```python
from build123d import *

# Parameters (mm, degrees)
ESQUISSE1_W        = 150
ESQUISSE1_H        = 50
ESQUISSE1_R        = 1
BOSS_EXTRU_4_DEPTH = 10
BOSS_EXTRU_5_DEPTH = 10


with BuildPart() as part:
    # Esquisse1 → Boss.-Extru.4 (new body)
    with BuildSketch(Plane(origin=(0, 0, -20), x_dir=(-1, 0, 0), z_dir=(0, 0, -1))):
        with Locations((11.141434162, -115.464178298)):
            Rectangle(ESQUISSE1_W, ESQUISSE1_H)
        with Locations((-43.858565838, -128.464178298)):
            Circle(ESQUISSE1_R, mode=Mode.SUBTRACT)
        with Locations((-43.858565838, -115.464178298)):
            Circle(ESQUISSE1_R, mode=Mode.SUBTRACT)
        with Locations((-33.858565838, -100.464178298)):
            Circle(ESQUISSE1_R, mode=Mode.SUBTRACT)
        with Locations((-8.858565838, -100.464178298)):
            Circle(ESQUISSE1_R, mode=Mode.SUBTRACT)
        with Locations((1.141434162, -115.464178298)):
            Circle(ESQUISSE1_R, mode=Mode.SUBTRACT)
        with Locations((1.141434162, -128.464178298)):
            Circle(ESQUISSE1_R, mode=Mode.SUBTRACT)
        with Locations((46.141434162, -123.464178298)):
            Circle(ESQUISSE1_R, mode=Mode.SUBTRACT)
        with Locations((46.141434162, -110.464178298)):
            Circle(ESQUISSE1_R, mode=Mode.SUBTRACT)
        with Locations((61.141434162, -100.464178298)):
            Circle(ESQUISSE1_R, mode=Mode.SUBTRACT)
        with Locations((76.141434162, -110.464178298)):
            Circle(ESQUISSE1_R, mode=Mode.SUBTRACT)
        with Locations((76.141434162, -123.464178298)):
            Circle(ESQUISSE1_R, mode=Mode.SUBTRACT)
    extrude(amount=BOSS_EXTRU_4_DEPTH)

    # Esquisse3 → Boss.-Extru.5 (add)
    with BuildSketch(Plane.XY.offset(-20)):
        Polygon((-1.141434162, -100.464178298), (-1.141434162, -90.464178298), (-21.141434162, -90.464178298), (-21.141434162, -140.464178298), (-11.141434162, -140.464178298), (-11.141434162, -100.464178298), align=None)
        Polygon((63.858565838, -140.464178298), (63.858565838, -90.464178298), (43.858565838, -90.464178298), (43.858565838, -100.464178298), (53.858565838, -100.464178298), (53.858565838, -140.464178298), align=None)
    extrude(amount=BOSS_EXTRU_5_DEPTH)


solid = part.part
```
Design review of the part built by this model. Coordinates are the model's own, in mm. A direction names the side the tool comes from. Coordinates: 2 decimals unless noted, no trailing zeros. Write each loop counter-clockwise with the first axis right and the second up, starting at its lowest first coordinate (ties: lowest second). Pieces come first, ordered by that corner, then holes.
1) Add section D-D (y = -107.5). Write out the cut boundary in (x, z), plus the area to 3 significant figures.
2) To check wall thickness, follow L1, parallel to X at y = -137.5, z = -19; L2, parallel to X at y = -92.5, z = -19.5; L3, parallel to Y at x = 53, z = -19.25. State the ranges of each line that lie inside material, in increasing order.
3) Add section A-A (z = -16.25). Write out the cut boundary in (x, y), plus the area to 3 significant figures.
4) Add section C-C (x = -6). Write out the cut boundary in (y, z), plus the area to 3 significant figures.
5) Add section B-B (y = -95). Write out the cut boundary in (x, z), plus the area to 3 significant figures.
6) Insertion check: pin 1 (11 mm diameter, centred on x = -5, z = -17, fed in from -Y); pin 2 (3 mm diameter, centred on x = -46.14, y = -123.46, fed in from +Z); pin 3 (5 mm diameter, centred on y = -127.5, z = -17, fed in from -X). Each pin has a flat end and moves straight along its axis. Give the tip position at first contact, or say it passes through.
7) Mouldability with a two-part tool opening along X and no side actions: class faces 1 (the flat face through (-21.141, -115, -15)), 2 (the flat face through (-1.141, -96, -15)), 3 (the flat face through (43.859, -95, -15)), 4 (the flat face through (-14, -110, -10)) as +X half, -X half, draft (parallel to the pull), parting line (faces both ways), or undercut.
8) Machinability: for faces 5 (the flat face through (-10, -90.464, -22)), 6 (the flat face through (-11.141, -121, -15)), 7 (the flat face through (-53, -115, -20)), which of the approach directions +Z, -Z, +X, -X, +Y, -Y give a long, thin tool a straight path to every point of the face, cutting with its end or side? Answer none if there is none.
Check result:
1. outline: (-86.14, -30) - (63.86, -30) - (63.86, -10) - (53.86, -10) - (53.86, -20) - (-11.14, -20) - (-11.14, -10) - (-21.14, -10) - (-21.14, -20) - (-86.14, -20) - close
1. area: 1,700 mm2
2. L1: x = -21.14 to -11.14, 53.86 to 63.86
2. L2: x = -21.14 to -1.14, 43.86 to 63.86
2. L3: y = -100.46 to -90.46
3. outline: (-21.14, -140.46) - (-11.14, -140.46) - (-11.14, -100.46) - (-1.14, -100.46) - (-1.14, -90.46) - (-21.14, -90.46) - close; (43.86, -100.46) - (53.86, -100.46) - (53.86, -140.46) - (63.86, -140.46) - (63.86, -90.46) - (43.86, -90.46) - close
3. area: 1,200 mm2
4. outline: (-140.46, -30) - (-90.46, -30) - (-90.46, -10) - (-100.46, -10) - (-100.46, -20) - (-140.46, -20) - close
4. area: 600 mm2
5. outline: (-86.14, -30) - (63.86, -30) - (63.86, -10) - (43.86, -10) - (43.86, -20) - (-1.14, -20) - (-1.14, -10) - (-21.14, -10) - (-21.14, -20) - (-86.14, -20) - close
5. area: 1,900 mm2
6. pin 1: stops at y = -140.46
6. pin 2: stops at z = -20
6. pin 3: stops at x = -21.14
7. face 1: -X half
7. face 2: undercut
7. face 3: undercut
7. face 4: draft
8. face 5: +Z, -Z, +X, -X, +Y
8. face 6: +Z, -Y
8. face 7: +Z, -X, +Y, -Y
